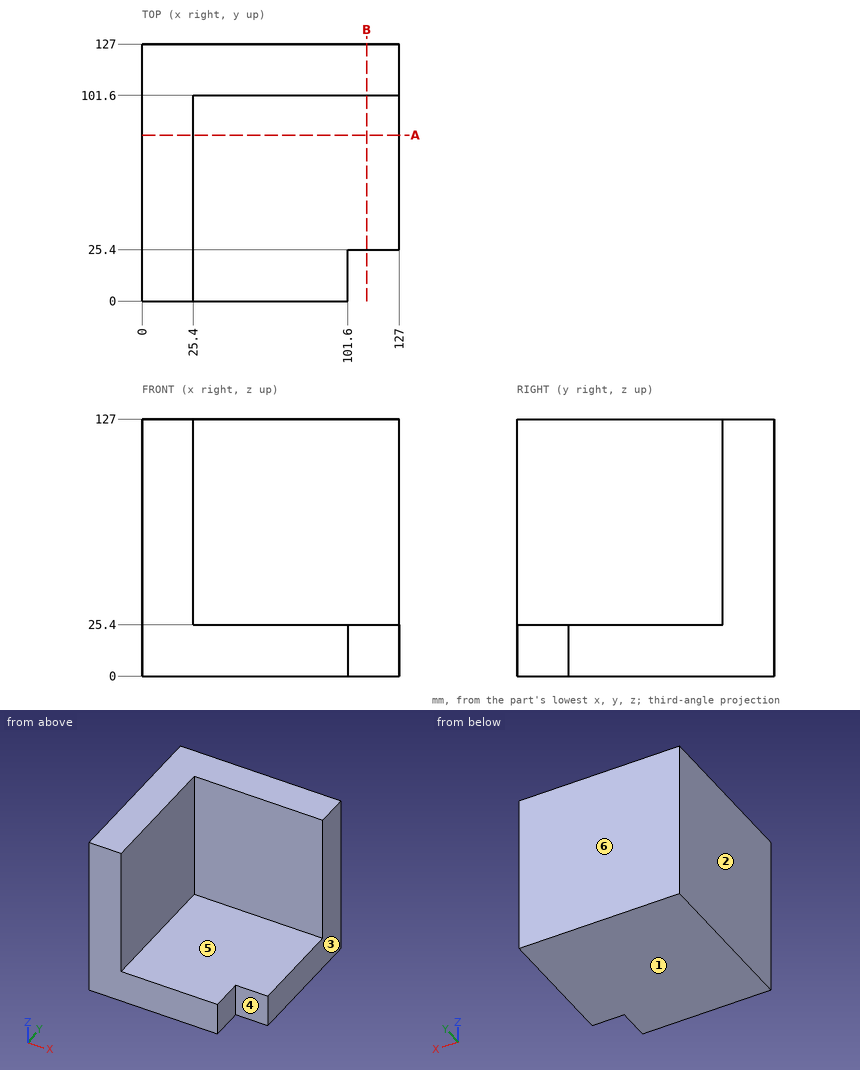
Geometry: see drawing. Coordinates: mm, zero at the bounding-box minimum. A direction names the side the tool comes from. Give positions to 0.01 mm unless a question says otherwise; leave off trailing zeros. Order: outer loops, then holes, each group sorted by start corner. A loop starts at its lowest first (then second) coordinate and runs counter-clockwise, first axis right, second up. Notation, with made-up numbers: (39, -13) - (50, -13) arc R17 ccw to (50, 4) - close; hole circle Ø7 at (-2.75, 75). An arc over 180 degrees is marked (long way). Use CSV: the item, a comma, the result in double quotes.
1. Contact query for flat-ended pins moving along their axis: pin 1 (12 mm diameter, centred on y = 68.5, z = 55.5, fed in from +X); pin 2 (1.5 mm diameter, centred on x = 45.5, z = 36, fed in from -Y); pin 3 (12 mm diameter, centred on x = 92, y = 68.5, fed in from +Z). Output: stop coordinate, or through.
Answers below:
pin 1,"x = 25.4"
pin 2,"y = 101.6"
pin 3,"z = 25.4"
2. Section query A-A (y = 82). Output: boundary loops of the cut face in (x, z), plus the area to 3 significant figures.
Answers below:
outline,"(0, 0) - (127, 0) - (127, 25.4) - (25.4, 25.4) - (25.4, 127) - (0, 127) - close"
area,"5,810 mm2"
3. Access query for the marked faces 4, 5 and 6. Directions: +Z, -Z, +X, -X, +Y, -Y. A direction counts if a zero-diameter tool reaches every point of the face in a straight line with its end or side. Return the directions, or none.
Answers below:
face 4,"+Z, -Z, +X, -Y"
face 5,"+Z, +X, -Y"
face 6,"+Z, -Z, +X, -X, +Y"
4. Material intervals for line 1 along Z through (x, y) = (65.5, 55); line 2 along Y through (x, z) = (74, 90), sorted ascending. Write a range as from..to.
Answers below:
line 1,"0..25.4"
line 2,"101.6..127"
5. Mould query, pull axis X, two halves, no side actions, for the marked faces 1, 2 and 3. Classes: +X half, -X half, draft (parallel to the pull), parting line (faces both ways), or undercut.
Answers below:
face 1,"draft"
face 2,"-X half"
face 3,"+X half"
6. Section query B-B (x = 111). Output: boundary loops of the cut face in (y, z), plus the area to 3 significant figures.
Answers below:
outline,"(25.4, 0) - (127, 0) - (127, 127) - (101.6, 127) - (101.6, 25.4) - (25.4, 25.4) - close"
area,"5,160 mm2"
